Read the model definition and answer for the solid it produces. Units are mm, in the model's axes. Face numbers are marked on the shaded views. A direction names the side the tool comes from. Coordinates: 2 decimals unless noted, no trailing zeros. Order: outer loops, then holes, each group sorted by start corner. A loop starts at its lowest first (then second) coordinate and runs counter-clockwise, first axis right, second up. Notation, with made-up numbers: (60.25, -4) - (105.25, -4) arc R24 cw to (105.25, 30) - close; hole circle Ø7 at (-6, 1.25). An arc over 180 degrees is marked (long way). Use one line per item in the form item = value. Start each with the question number.
from build123d import *

# Parameters (mm, degrees)
SKETCH1_W           = 80
SKETCH1_H           = 35
BOSS_EXTRUDE1_DEPTH = 1
SKETCH2_W           = 70
SKETCH2_H           = 24
BOSS_EXTRUDE2_DEPTH = 6
SKETCH3_W           = 44.648131597
SKETCH3_H           = 14.861449517
BOSS_EXTRUDE3_DEPTH = 3
SKETCH4_W           = 2
SKETCH4_H           = 14.195770454
CUT_EXTRUDE1_DEPTH  = 77.228769639
SKETCH5_W           = 3.954548799
SKETCH5_H           = 8.674494139
BOSS_EXTRUDE4_DEPTH = 1


with BuildPart() as part:
    # Sketch1 → Boss-Extrude1 (new body)
    with BuildSketch(Plane.XY):
        Rectangle(SKETCH1_W, SKETCH1_H)
    extrude(amount=BOSS_EXTRUDE1_DEPTH)

    # Sketch2 → Boss-Extrude2 (add)
    with BuildSketch(Plane.XY.offset(1)):
        Rectangle(SKETCH2_W, SKETCH2_H)
    extrude(amount=BOSS_EXTRUDE2_DEPTH)

    # Sketch3 → Boss-Extrude3 (add)
    with BuildSketch(Plane(origin=(0, 0, 0), x_dir=(-1, 0, 0), z_dir=(0, 0, -1))):
        with Locations((-13.90470384, -7.430724759)):
            Rectangle(SKETCH3_W, SKETCH3_H)
    extrude(amount=BOSS_EXTRUDE3_DEPTH)

    # Sketch4 → Cut-Extrude1 (cut, through all)
    with BuildSketch(Plane(origin=(36.228769639, 0, 0), x_dir=(0, 0, -1), z_dir=(1, 0, 0))):
        with Locations((1, -6.56356429)):
            Rectangle(SKETCH4_W, SKETCH4_H)
    extrude(amount=-CUT_EXTRUDE1_DEPTH, mode=Mode.SUBTRACT)

    # Sketch5 → Boss-Extrude4 (add)
    with BuildSketch(Plane(origin=(0, 0, -3), x_dir=(-1, 0, 0), z_dir=(0, 0, -1))):
        with Locations((-14.096052976, -7.845314553)):
            Rectangle(SKETCH5_W, SKETCH5_H)
    extrude(amount=BOSS_EXTRUDE4_DEPTH)


solid = part.part
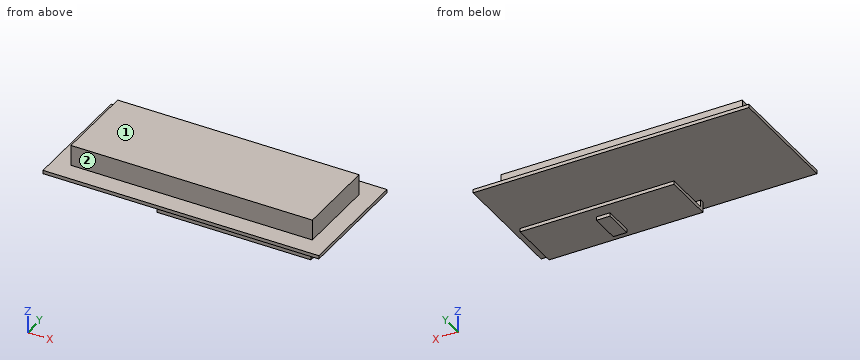
Q1. Consider probe 1 along Z at (x, y) = (31.5, -13.5); probe 2 along Z at (x, y) = (12, -0.5); probe 3 along Z at (x, y) = (-2, 1.5). Determine where each line is inside the solid, lowest interval first.
Q2. A cutting plane is placed at C-C (y = 6.5). Give the vertices of the cut face in (x, z).
Q3. A cutting plane is placed at A-A (y = -9.5). Give the vertices of the cut face in (x, z), then the cut area to 3 significant figures.
Q4. Given P1, Ø1.1, axis at x = 14, z = -3.5, coming from the +Y side; P2, Ø17.5, axis at x = -8, y = -4.5, coming from the -Z side; P3, Ø0.5, axis at x = 13.5, z = -3.5, coming from the -Y side, each flat-ended and moving along its own axis, determine where each tip first touches the part or whether it passes through.
Q5. Which of the six approach directions +Z, -Z, +X, -X, +Y, -Y give full straight-line access (tool end or side, diameter ignored) to the marked faces 1 and 2?
Q6. A cutting plane is placed at B-B (x = 24.5). Give the vertices of the cut face in (y, z).
Q7. A cutting plane is placed at D-D (z = 5.25). Give the vertices of the cut face in (x, y), then the cut area to 3 significant figures.
Result sheet:
q1.probe_1 = -3 to -2, 0 to 1
q1.probe_2 = -3 to -2, 0 to 7
q1.probe_3 = 0 to 7
q2.outline = (-40, 0) - (40, 0) - (40, 1) - (35, 1) - (35, 7) - (-35, 7) - (-35, 1) - (-40, 1) - close
q3.outline = (-40, 0) - (40, 0) - (40, 1) - (35, 1) - (35, 7) - (-35, 7) - (-35, 1) - (-40, 1) - close; (-8.42, -3) - (12.12, -3) - (12.12, -4) - (16.07, -4) - (16.07, -3) - (36.23, -3) - (36.23, -2) - (-8.42, -2) - close
q3.area = 549 mm^2
q4.P1 = 0
q4.P2 = -3
q4.P3 = -12.18
q5.face_1 = +Z, +X, -X, +Y, -Y
q5.face_2 = +Z, +X, -X, -Y
q6.outline = (-17.5, 0) - (-14.86, 0) - (-14.86, -3) - (0, -3) - (0, -2) - (-13.66, -2) - (-13.66, 0) - (17.5, 0) - (17.5, 1) - (12, 1) - (12, 7) - (-12, 7) - (-12, 1) - (-17.5, 1) - close
q7.outline = (-35, -12) - (35, -12) - (35, 12) - (-35, 12) - close
q7.area = 1,680 mm^2
